from build123d import *

# Parameters (mm, degrees)
SKETCH1_W           = 45
SKETCH1_H           = 6
BOSS_EXTRUDE1_DEPTH = 4
SKETCH2_R           = 1.65
CUT_EXTRUDE1_DEPTH  = 46.57411546
SKETCH4_W           = 14
SKETCH4_H           = 6
BOSS_EXTRUDE2_DEPTH = 4
SKETCH5_W           = 3
SKETCH5_H           = 6
CUT_EXTRUDE2_DEPTH  = 10
SKETCH6_R           = 1
CUT_EXTRUDE3_DEPTH  = 47.097722286
FILLET1_R           = 2
FILLET2_R           = 3
FILLET3_R           = 2
FILLET4_R           = 2


with BuildPart() as part:
    # Sketch1 → Boss-Extrude1 (new body)
    with BuildSketch(Plane(origin=(0, 0, 0), x_dir=(0, 0, -1), z_dir=(1, 0, 0))):
        with Locations((22.5, -3)):
            Rectangle(SKETCH1_W, SKETCH1_H)
    extrude(amount=BOSS_EXTRUDE1_DEPTH)

    # Sketch2 → Cut-Extrude1 (cut, through all)
    with BuildSketch(Plane(origin=(4, 0, 0), x_dir=(0, 0, -1), z_dir=(1, 0, 0))):
        with Locations((5, -3)):
            Circle(SKETCH2_R)
    extrude(amount=-CUT_EXTRUDE1_DEPTH, mode=Mode.SUBTRACT)

    # Sketch4 → Boss-Extrude2 (add)
    with BuildSketch(Plane.ZY):
        with Locations((-38, -3)):
            Rectangle(SKETCH4_W, SKETCH4_H)
    extrude(amount=BOSS_EXTRUDE2_DEPTH)

    # Sketch5 → Cut-Extrude2 (cut)
    with BuildSketch(Plane(origin=(0, 0, -45), x_dir=(-1, 0, 0), z_dir=(0, 0, -1))):
        with Locations((0, -3)):
            Rectangle(SKETCH5_W, SKETCH5_H)
    extrude(amount=-CUT_EXTRUDE2_DEPTH, mode=Mode.SUBTRACT)

    # Sketch6 → Cut-Extrude3 (cut, through all)
    with BuildSketch(Plane.ZY.offset(4)):
        with Locations((-41.5, -3)):
            Circle(SKETCH6_R)
    extrude(amount=-CUT_EXTRUDE3_DEPTH, mode=Mode.SUBTRACT)

    # Fillet1
    fillet1_edges = [part.edges().sort_by_distance(p)[0] for p in [
        (2, 0, 0),
        (2.75, 0, -45),
        (2.75, -6, -45),
        (2, -6, 0),
    ]]
    fillet(fillet1_edges, radius=FILLET1_R)

    # Fillet2
    fillet2_edges = [part.edges().sort_by_distance(p)[0] for p in [
        (0, -3, -31),
    ]]
    fillet(fillet2_edges, radius=FILLET2_R)

    # Fillet3
    fillet3_edges = [part.edges().sort_by_distance(p)[0] for p in [
        (-4, -3, -31),
    ]]
    fillet(fillet3_edges, radius=FILLET3_R)

    # Fillet4
    fillet4_edges = [part.edges().sort_by_distance(p)[0] for p in [
        (-2.75, 0, -45),
        (-2.75, -6, -45),
    ]]
    fillet(fillet4_edges, radius=FILLET4_R)


solid = part.part
Input: part model. Units: mm. Frame: model coordinates. A direction names the side the tool comes from. Coordinates: 2 decimals unless noted, no trailing zeros. Loops run counter-clockwise (first coordinate to the right, second up) from the corner with the lowest first, then second, coordinate; pieces in that order, holes last.
(1) Set-up query: faces 5 (the face through (0, -3, -35)), 6 (the face through (0, -3, -14)), 7 (the face through (2.03, -5.43, -0.6)). Return all of +Z, -Z, +X, -X, +Y, -Y with unobstructed straight access to the full face (end or side cutting, diameter ignored); none if empty.
(2) Pull-direction query (Z, two-part tool) for faces 1 (the face through (-2.768, -2.7, -40.546)), 2 (the face through (-2.73, -0.6, -44.43)), 3 (the face through (-1.5, -3, -40)), 4 (the face through (2.732, -2.7, -40.546)); classes: released by +Z, released by -Z, zero draft, split by the parting line, or undercut.
(3) Section A-A on z = -5. Return the cut outline in (x, y), then the cut area to 3 significant figures.
(4) Section C-C on y = -3. Count the separate pieces of the cut face and the enclosed holes in it, then the cut area to 3 significant figures.
(5) Material intervals for probe 1 along X at (y, z) = (-2.5, -43); probe 2 along X at (y, z) = (-4, -13); probe 3 along Z at (x, y) = (3.25, -4.25), sorted ascending.
(6) First-contact query: pin 1 Ø3 at (y, z) = (-3, -10) entering from -X; pin 2 Ø1.5 at (x, y) = (0.5, -1.5) entering from -Z. Flat tips, straight axial feed; report the tip coordinate or a pass-through.
(7) Section B-B on z = -41.5. Return the cut outline in (x, y), then the cut area to 3 significant figures.
(8) Section D-D on x = -0.75. Return the cut outline in (y, z).
Data:
1. face 5: -Z, +Y, -Y
1. face 6: +Z, -X, +Y, -Y
1. face 7: +Z, +X, -X, -Y
2. face 1: undercut
2. face 2: released by -Z
2. face 3: zero draft
2. face 4: undercut
3. outline: (0, -6) - (4, -6) - (4, -4.65) - (0, -4.65) - close; (0, -1.35) - (4, -1.35) - (4, 0) - (0, 0) - close
3. area: 10.8 mm2
4. separate pieces: 4
4. enclosed holes: 0
4. area: 184 mm2
5. probe 1: x = -4 to -1.5, 1.5 to 4
5. probe 2: x = 0 to 4
5. probe 3: z = -44.98 to -6.08, -3.92 to -0.02
6. pin 1: stops at x = 0
6. pin 2: stops at z = -35
7. outline: (-4, -6) - (-1.5, -6) - (-1.5, -4) - (-4, -4) - close; (-4, -2) - (-1.5, -2) - (-1.5, 0) - (-4, 0) - close; (1.5, -6) - (4, -6) - (4, -4) - (1.5, -4) - close; (1.5, -2) - (4, -2) - (4, 0) - (1.5, 0) - close
7. area: 20.0 mm2
8. outline: (-6, -35) - (0, -35) - (0, -29.98) - (-6, -29.98) - close
